from build123d import *

# Parameters (mm, degrees)
F0_R     = 5.55625
F1_DEPTH = 1.5748
F2_R     = 26.9875
F3_DEPTH = 15.8877
F4_R     = 16.4211
F5_DEPTH = 11.1125
F6_R     = 9.525
F7_DEPTH = 28.575


with BuildPart() as f1:
    # F0 (on Front) → F1 (new body)
    with BuildSketch(Plane.XZ):
        with BuildLine():
            Line((28.575, 19.05), (9.185667, 47.528893))
            ThreePointArc((9.185667, 47.528893), (0, 52.3875), (-9.185667, 47.528893))
            Line((-9.185667, 47.528893), (-28.575, 19.05))
            Line((-28.575, 19.05), (-28.575, -19.05))
            Line((-28.575, -19.05), (-9.185667, -47.528893))
            ThreePointArc((-9.185667, -47.528893), (0, -52.3875), (9.185667, -47.528893))
            Line((9.185667, -47.528893), (28.575, -19.05))
            Line((28.575, -19.05), (28.575, 19.05))
        make_face()
        with Locations((0, -41.275)):
            Circle(F0_R, mode=Mode.SUBTRACT)
        with Locations((0, 41.275)):
            Circle(F0_R, mode=Mode.SUBTRACT)
    extrude(amount=F1_DEPTH)

    # F2 (on face) → F3 (join)
    with BuildSketch(Plane.XZ.offset(1.5748)):
        Circle(F2_R)
    extrude(amount=F3_DEPTH)

    # F4 (on face) → F5 (join)
    with BuildSketch(Plane.XZ.offset(17.4625)):
        Circle(F4_R)
    extrude(amount=F5_DEPTH)

    # F6 (on face) → F7 (cut, through all)
    with BuildSketch(Plane.XZ.offset(28.575)):
        Circle(F6_R)
    extrude(amount=-F7_DEPTH, mode=Mode.SUBTRACT)


solid = f1.part
Source: CAD feature listing. Evaluate the final solid. Frame: model axes, mm. A direction names the side the tool comes from. Coordinates: 2 decimals unless noted, no trailing zeros. Write each loop counter-clockwise with the first axis right and the second up, starting at its lowest first coordinate (ties: lowest second). Pieces come first, ordered by that corner, then holes. Notation, with made-up numbers: M 34,52.5 L 83,52.5 A24 cw 83,69.5 Z; hole C 13,54.5 d8. An arc over 180 degrees is marked long. Use a Markdown table: item, result.
1) Mould query, pull axis X, two halves, no side actions, for faces 3 (the flat face through (19.016, -0.776, 33.09)), 4 (the cylindrical face through (-19.89, -9.41, 18.24)), 5 (the cylindrical face through (-7.559, -14.488, -5.796)), 6 (the cylindrical face through (2.99, -0.78, 45.96)). Classes: pulls with the +X half, pulls with the -X half, needs draft (parallel to the pull), parting line crosses it, or undercut.
Conclusion:
| item | result |
|---|---|
| face 3 | pulls with the +X half |
| face 4 | parting line crosses it |
| face 5 | undercut |
| face 6 | undercut |
2) Ray query, L1, parallel to Z at x = 0, y = -0.85 (1 decimal); L2, parallel to Y at x = -5.5, z = -27.5; L3, parallel to X at y = -10.75, z = 6.5. Return the intervals inside material, ascending.
Conclusion:
| item | result |
|---|---|
| L1 | z = -52.4 to -46.8, -35.7 to -9.5, 9.5 to 35.7, 46.8 to 52.4 |
| L2 | y = -1.57 to 0 |
| L3 | x = -26.19 to -6.96, 6.96 to 26.19 |
3) Section B-B, the plane x = 0. Output: boundary loops of the cut face in (y, z) (1 decimal).
Conclusion:
| item | result |
|---|---|
| outline | M -28.6,-16.4 L -17.5,-16.4 L -17.5,-27 L -1.6,-27 L -1.6,-35.7 L 0,-35.7 L 0,-9.5 L -28.6,-9.5 Z; M -28.6,9.5 L 0,9.5 L 0,35.7 L -1.6,35.7 L -1.6,27 L -17.5,27 L -17.5,16.4 L -28.6,16.4 Z; M -1.6,-52.4 L 0,-52.4 L 0,-46.8 L -1.6,-46.8 Z; M -1.6,46.8 L 0,46.8 L 0,52.4 L -1.6,52.4 Z |
4) Section D-D, the plane z = -44.5. Output: boundary loops of the cut face in (x, y).
Conclusion:
| item | result |
|---|---|
| outline | M -11.25,-1.57 L -4.52,-1.57 L -4.52,0 L -11.25,0 Z; M 4.52,-1.57 L 11.25,-1.57 L 11.25,0 L 4.52,0 Z |
5) First-contact query: pin 1 Ø10 at (x, z) = (0, 41.275) entering from +Y; pin 2 Ø1 at (x, z) = (-15, 8) entering from -Y; pin 3 Ø13 at (x, z) = (0, -41.275) entering from -Y; pin 4 Ø1 at (y, z) = (-14.5, 9.5) entering from +X. Flat tips, straight axial feed; report the tip coordinate or a pass-through.
Conclusion:
| item | result |
|---|---|
| pin 1 | passes through |
| pin 2 | stops at y = -17.46 |
| pin 3 | stops at y = -1.57 |
| pin 4 | stops at x = 25.44 |
6) Section A-A, the plane z = 0. Output: boundary loops of the cut face in (x, y) (1 decimal), then the cut area to 3 significant figures.
Conclusion:
| item | result |
|---|---|
| outline | M -28.6,-1.6 L -27,-1.6 L -27,-17.5 L -16.4,-17.5 L -16.4,-28.6 L -9.5,-28.6 L -9.5,0 L -28.6,0 Z; M 9.5,-28.6 L 16.4,-28.6 L 16.4,-17.5 L 27,-17.5 L 27,-1.6 L 28.6,-1.6 L 28.6,0 L 9.5,0 Z |
| area | 768 mm^2 |
7) Section C-C, the plane y = -23. Output: boundary loops of the cut face in (x, z) (3 decimals), then the cut area to 3 significant figures.
Conclusion:
| item | result |
|---|---|
| outline | C 0,0 d32.842; hole C 0,0 d19.05 |
| area | 562 mm^2 |
8) Reachability of faces 1 (the flat face through (7, -28.575, -7)), 2 (the flat face through (12, -17.463, -12)) from +Z, -Z, +X, -X, +Y, -Y: full face, straight path, thin tool, end or side. Return the list, or none.
Conclusion:
| item | result |
|---|---|
| face 1 | +Z, -Z, +X, -X, -Y |
| face 2 | -Y |
